Source: CAD feature listing. Evaluate the final solid. Frame: model axes, mm. A direction names the side the tool comes from. Coordinates: 2 decimals unless noted, no trailing zeros. Write each loop counter-clockwise with the first axis right and the second up, starting at its lowest first coordinate (ties: lowest second). Pieces come first, ordered by that corner, then holes. Notation, with made-up numbers: (16, -18.75) -> (72, -18.75) arc R22 ccw to (72, 5.25) -> close; hole circle Ø1 at (-7.5, -5.5). An arc over 180 degrees is marked (long way). One line per item, written item: value. Start each with the question number.
1. Section query A-A, the plane y = 2.75. Output: boundary loops of the cut face in (x, z).
2. Line query: line 1 (Z direction, x = 57.5, y = 6.75); line 2 (X direction, y = 4, z = 4.5); line 3 (Z direction, x = -4, y = 4.75). Output: solid intervals per line, ascending.
3. Section query B-B, the plane z = -6. Output: boundary loops of the cut face in (x, y), and give its area (3 significant figures).
4. First-contact query: P1, Ø8, axis at x = -53.18, z = 35.61, coming from the -Y side; P2, Ø1.5, axis at x = 94.5, y = 5.5, coming from the -Z side; P3, Ø1.5, axis at x = -4, z = 36, coming from the +Y side. Flat tips, straight axial feed; report the tip coordinate or a pass-through.
5. Mould query, pull axis X, two halves, no side actions, for faces 4 (the flat face through (-28, 3, -31.895)), 5 (the flat face through (14.318, 3, 1)), 6 (the flat face through (-3, 4, 36)). Classes: released by +X, released by -X, zero draft, split by the parting line, or undercut.
6. Access query for faces 1 (the flat face through (65, 3, 33.105)), 2 (the flat face through (0, 0, 53)), 3 (the cylindrical face through (-55.68, 5.52, -14.5)). Directions: +Z, -Z, +X, -X, +Y, -Y. A direction counts if a zero-diameter tool reaches every point of the face in a straight line with its end or side. Return the directions, or none.
7. Section query C-C, the plane x = 92.5. Output: boundary loops of the cut face in (y, z).
from build123d import *

# Parameters (mm, degrees)
BOSS_EXTRUDE1_DEPTH = 7
SKETCH2_R           = 2.5
CUT_EXTRUDE2_DEPTH  = 3


with BuildPart() as part:
    # Sketch1 → Boss-Extrude1 (new body)
    with BuildSketch(Plane(origin=(0, 0, 0), x_dir=(1, 0, 0), z_dir=(0, 1, 0))):
        Polygon((14.318293597, 31.894904459), (-70.681706403, 31.894904459), (-70.681706403, -108.105095541), (114.318293597, -108.105095541), (114.318293597, -33.105095541), (14.318293597, -33.105095541), align=None)
    extrude(amount=BOSS_EXTRUDE1_DEPTH)

    # Sketch2 → Cut-Extrude2 (cut)
    with BuildSketch(Plane(origin=(0, 7, 0), x_dir=(1, 0, 0), z_dir=(0, 1, 0))):
        with Locations((-53.181706403, 14.394904459)):
            Circle(SKETCH2_R)
        with Locations((-3.181706403, 14.394904459)):
            Circle(SKETCH2_R)
        with Locations((-3.181706403, -35.605095541)):
            Circle(SKETCH2_R)
        with Locations((-53.181706403, -35.605095541)):
            Circle(SKETCH2_R)
    extrude(amount=-CUT_EXTRUDE2_DEPTH, mode=Mode.SUBTRACT)


solid = part.part
Computed values:
1. outline: (-70.68, -31.89) -> (14.32, -31.89) -> (14.32, 33.11) -> (114.32, 33.11) -> (114.32, 108.11) -> (-70.68, 108.11) -> close
2. line 1: z = 33.11 to 108.11
2. line 2: x = -70.68 to 14.32
2. line 3: z = -31.89 to -16.76, -12.03 to 33.24, 37.97 to 108.11
3. outline: (-70.68, 0) -> (14.32, 0) -> (14.32, 7) -> (-70.68, 7) -> close
3. area: 595 mm²
4. P1: stops at y = 0
4. P2: stops at z = 33.11
4. P3: stops at y = 4
5. face 4: zero draft
5. face 5: released by +X
5. face 6: undercut
6. face 1: -Z, +X, +Y, -Y
6. face 2: +Z, -Z, +X, -X, -Y
6. face 3: +Y
7. outline: (0, 33.11) -> (7, 33.11) -> (7, 108.11) -> (0, 108.11) -> close
